Could you check a few things on this drawing? It's one solid part, dimensions in mm from its lowest x, y, z. A direction names the side the tool comes from. Coordinates: 2 decimals unless noted, no trailing zeros. Order: outer loops, then holes, each group sorted by start corner. A loop starts at its lowest first (then second) coordinate and runs counter-clockwise, first axis right, second up.
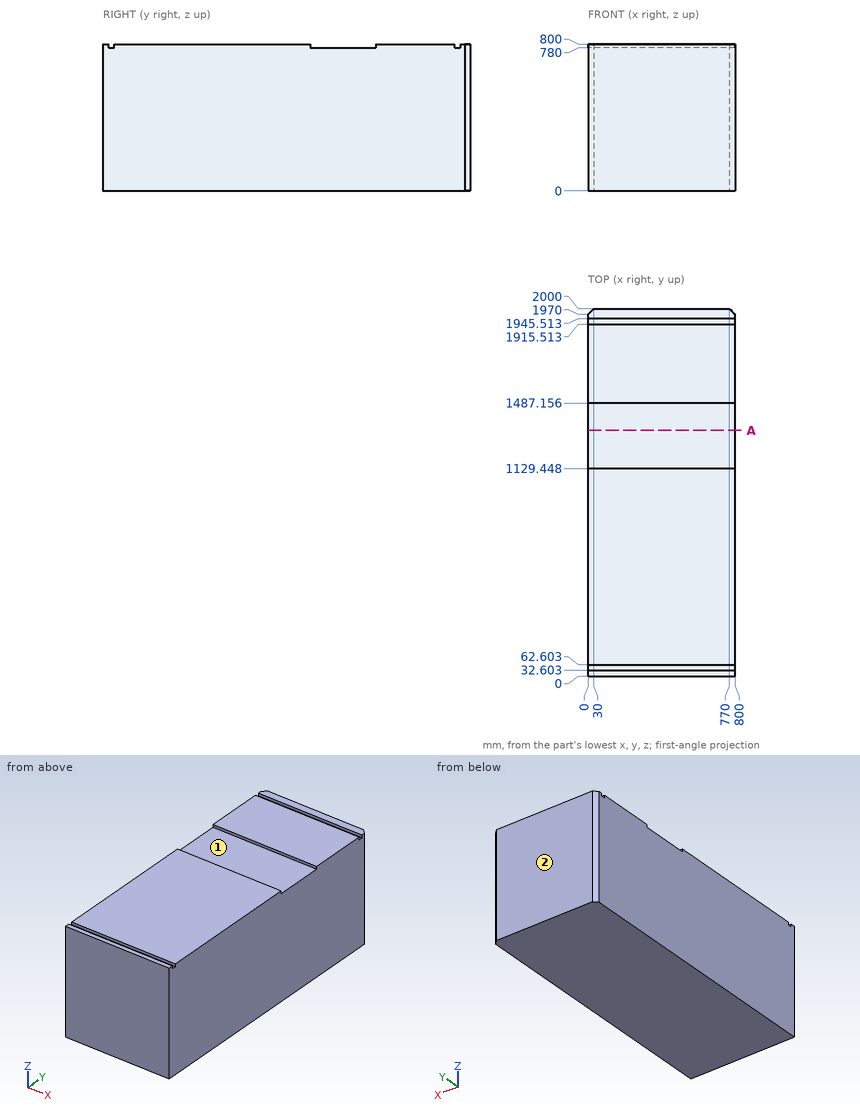
1. Imagine slicing it at A-A on y = 1337.5. Please give me the cut outline in (x, z).
Completed:
outline: (0, 0) - (800, 0) - (800, 780) - (0, 780) - close
2. Please list where this line runs through material, in increasing order: probe 1 along Z at (x, y) = (200.5, 1168).
Completed:
probe 1: z = 0 to 780
3. On a 3-axis mill with a long thin cutter (end or side, diameter ignored), from which of +Z, -Z, +X, -X, +Y, -Y can I reach the whole of each face in a straight line? I mean the marked faces 1 and 2. Say none if no direction works.
Completed:
face 1: +Z, +X, -X
face 2: +Z, -Z, +X, -X, +Y
4. I'm going to push a flat-ended pin straight in: pin 1 (24 mm diameter, centred on x = 281.5, y = 1931.5, fed in from +Z). Where does the tip first touch, or does it pass through?
Completed:
pin 1: stops at z = 780
